from build123d import *

# Parameters (mm, degrees)
SKETCH1_R           = 1.5
BOSS_EXTRUDE2_DEPTH = 3.175


with BuildPart() as part:
    # Sketch1 → Boss-Extrude2 (new body)
    with BuildSketch(Plane(origin=(0, 0, 0), x_dir=(1, 0, 0), z_dir=(0, 1, 0))):
        with BuildLine():
            ThreePointArc((35.49727084, -66.067721036), (0, 75), (-35.49727084, -66.067721036))
            ThreePointArc((-35.49727084, -66.067721036), (-33.357679643, -66.33740492), (-31.589980006, -65.102164912))
            ThreePointArc((-31.589980006, -65.102164912), (0, -48.302004425), (31.589980006, -65.102164912))
            ThreePointArc((31.589980006, -65.102164912), (33.357679643, -66.33740492), (35.49727084, -66.067721036))
        make_face()
        with Locations((-13.608916499, -21.183093811)):
            Circle(SKETCH1_R, mode=Mode.SUBTRACT)
        with Locations((-46.011477091, 28.075890486)):
            Circle(SKETCH1_R, mode=Mode.SUBTRACT)
        with Locations((13.608916499, -21.183093811)):
            Circle(SKETCH1_R, mode=Mode.SUBTRACT)
        with Locations((23.852486199, -41.694616163)):
            Circle(SKETCH1_R, mode=Mode.SUBTRACT)
        with Locations((-42.910067426, 11.1)):
            Circle(SKETCH1_R, mode=Mode.SUBTRACT)
        with Locations((-42.910067426, -11.1)):
            Circle(SKETCH1_R, mode=Mode.SUBTRACT)
        with Locations((-11.160067426, -11.1)):
            Circle(SKETCH1_R, mode=Mode.SUBTRACT)
        with Locations((-11.160067426, 11.1)):
            Circle(SKETCH1_R, mode=Mode.SUBTRACT)
        with Locations((11.160067426, 11.1)):
            Circle(SKETCH1_R, mode=Mode.SUBTRACT)
        with Locations((11.160067426, -11.1)):
            Circle(SKETCH1_R, mode=Mode.SUBTRACT)
        with Locations((42.910067426, -11.1)):
            Circle(SKETCH1_R, mode=Mode.SUBTRACT)
        with Locations((42.910067426, 11.1)):
            Circle(SKETCH1_R, mode=Mode.SUBTRACT)
        with Locations((-23.852486199, -41.694616163)):
            Circle(SKETCH1_R, mode=Mode.SUBTRACT)
        with Locations((19.397913834, 18.186588214)):
            Circle(SKETCH1_R, mode=Mode.SUBTRACT)
        with Locations((-40.277379234, -25.14022965)):
            Circle(SKETCH1_R, mode=Mode.SUBTRACT)
        with Locations((40.277379234, -25.14022965)):
            Circle(SKETCH1_R, mode=Mode.SUBTRACT)
        with Locations((-22.416161975, 64.096715224)):
            Circle(SKETCH1_R, mode=Mode.SUBTRACT)
        with Locations((22.416161975, 64.096715224)):
            Circle(SKETCH1_R, mode=Mode.SUBTRACT)
        with Locations((26.163250867, 37.1696126)):
            Circle(SKETCH1_R, mode=Mode.SUBTRACT)
        with Locations((46.011477091, 28.075890486)):
            Circle(SKETCH1_R, mode=Mode.SUBTRACT)
        with Locations((10.027203595, 39.91869143)):
            Circle(SKETCH1_R, mode=Mode.SUBTRACT)
        with Locations((0, -39.659190322)):
            Circle(SKETCH1_R, mode=Mode.SUBTRACT)
        with Locations((-10.027203595, 39.91869143)):
            Circle(SKETCH1_R, mode=Mode.SUBTRACT)
        with Locations((-34.69516474, -58.122990171)):
            Circle(SKETCH1_R, mode=Mode.SUBTRACT)
        with Locations((-34.69516474, 58.122990171)):
            Circle(SKETCH1_R, mode=Mode.SUBTRACT)
        with Locations((34.69516474, -58.122990171)):
            Circle(SKETCH1_R, mode=Mode.SUBTRACT)
        with Locations((0, 15.543589551)):
            Circle(SKETCH1_R, mode=Mode.SUBTRACT)
        with Locations((-26.163250867, 37.1696126)):
            Circle(SKETCH1_R, mode=Mode.SUBTRACT)
        with Locations((-19.397913834, 18.186588214)):
            Circle(SKETCH1_R, mode=Mode.SUBTRACT)
        with Locations((34.69516474, 58.122990171)):
            Circle(SKETCH1_R, mode=Mode.SUBTRACT)
        with BuildLine():
            Line((53.410067426, -34), (53.410067426, 34))
            ThreePointArc((53.410067426, 34), (53.556514035, 34.353553391), (53.910067426, 34.5))
            Line((53.910067426, 34.5), (63.910067426, 34.5))
            ThreePointArc((63.910067426, 34.5), (64.263620817, 34.353553391), (64.410067426, 34))
            Line((64.410067426, 34), (64.410067426, -34))
            ThreePointArc((64.410067426, -34), (64.263620817, -34.353553391), (63.910067426, -34.5))
            Line((63.910067426, -34.5), (53.910067426, -34.5))
            ThreePointArc((53.910067426, -34.5), (53.556514035, -34.353553391), (53.410067426, -34))
        make_face(mode=Mode.SUBTRACT)
        with BuildLine():
            Line((-63.910067426, -34.5), (-53.910067426, -34.5))
            ThreePointArc((-53.910067426, -34.5), (-53.556514035, -34.353553391), (-53.410067426, -34))
            Line((-53.410067426, -34), (-53.410067426, 34))
            ThreePointArc((-53.410067426, 34), (-53.556514035, 34.353553391), (-53.910067426, 34.5))
            Line((-53.910067426, 34.5), (-63.910067426, 34.5))
            ThreePointArc((-63.910067426, 34.5), (-64.263620817, 34.353553391), (-64.410067426, 34))
            Line((-64.410067426, 34), (-64.410067426, -34))
            ThreePointArc((-64.410067426, -34), (-64.263620817, -34.353553391), (-63.910067426, -34.5))
        make_face(mode=Mode.SUBTRACT)
        with BuildLine():
            ThreePointArc((-5.853899988, 64.744946271), (0.003726822, 68.153564176), (5.857575472, 64.738461857))
            ThreePointArc((5.857575472, 64.738461857), (10.16, 61.422565207), (5.857575472, 58.106668557))
            ThreePointArc((5.857575472, 58.106668557), (0.003726822, 54.691566239), (-5.853899988, 58.100184144))
            ThreePointArc((-5.853899988, 58.100184144), (-10.167207264, 61.422565207), (-5.853899988, 64.744946271))
        make_face(mode=Mode.SUBTRACT)
    extrude(amount=BOSS_EXTRUDE2_DEPTH)


solid = part.part
Check sheet for the modelled part. Datum: model origin and axes. Units: mm. A direction names the side the tool comes from. Round coordinates to 2 decimals unless told otherwise and drop trailing zeros. Order: outer loops, then holes, each group sorted by start corner. A loop starts at its lowest first (then second) coordinate and runs counter-clockwise, first axis right, second up.
(1) Go/stop test with flat-tipped pins: P1, Ø1, axis at y = 0.5, z = -12.5, coming from the -X side; P2, Ø1.6, axis at y = 2.5, z = -13, coming from the +X side; P3, Ø1, axis at x = 53, y = 1, coming from the +Z side. Record where each tip stops, or that it passes through.
(2) Access from +Z, -Z, +X, -X, +Y, -Y to the whole of each face (thin tool, end or side, straight path). Record for faces 1 (the cylindrical face through (-0.096, 1.565, -68.153)), 2 (the cylindrical face through (-0.521, 1.565, 48.306)).
(3) Cross-section at D-D, the plane y = 1. State how many separate pieces and enclosed holes the cut face has, and give its area (3 significant figures).
(4) Cross-section at C-C, the plane z = 32. Enter the section's corners in (x, y) (3 decimals).
(5) Draft check along X on faces 3 (the flat face through (-1, 0, -5)), 4 (the cylindrical face through (-10.166, 1.565, -61.335)), 5 (the cylindrical face through (2.78, 1.57, -74.95)). Enter one of: pulls with the +X half, pulls with the -X half, needs draft (parallel to the pull), parting line crosses it, or undercut.
(6) Scan lines: probe 1 along X at (y, z) = (3.05, -9); probe 2 along X at (y, z) = (1.8, -2.5); probe 3 along X at (y, z) = (1.1, -59). Record each from-to range of solid material in increasing order.
(7) Cross-section at A-A, the plane z = 0. Enter the section's corners in (x, y) (3 decimals), and give its area (3 significant figures).
(8) Cross-section at B-B, the plane x = -56. Enter the section's corners in (y, z) (3 decimals).
Check sheet entries:
1. P1: stops at x = -74.03
1. P2: stops at x = 74
1. P3: stops at z = 53.56
2. face 1: +Y, -Y
2. face 2: +Z, +Y, -Y
3. separate pieces: 1
3. enclosed holes: 33
3. area: 14,500 mm2
4. outline: (-67.831, 0) - (-64.41, 0) - (-64.41, 3.175) - (-67.831, 3.175) - close; (-53.41, 0) - (53.41, 0) - (53.41, 3.175) - (-53.41, 3.175) - close; (64.41, 0) - (67.831, 0) - (67.831, 3.175) - (64.41, 3.175) - close
5. face 3: needs draft
5. face 4: undercut
5. face 5: parting line crosses it
6. probe 1: x = -74.46 to -64.41, -53.41 to 53.41, 64.41 to 74.46
6. probe 2: x = -74.96 to -64.41, -53.41 to 53.41, 64.41 to 74.96
6. probe 3: x = -46.3 to -35.91, -33.48 to -9.17, 9.16 to 33.48, 35.91 to 46.3
7. outline: (-75, 0) - (-64.41, 0) - (-64.41, 3.175) - (-75, 3.175) - close; (-53.41, 0) - (53.41, 0) - (53.41, 3.175) - (-53.41, 3.175) - close; (64.41, 0) - (75, 0) - (75, 3.175) - (64.41, 3.175) - close
7. area: 406 mm2
8. outline: (0, -49.89) - (3.175, -49.89) - (3.175, -34.5) - (0, -34.5) - close; (0, 34.5) - (3.175, 34.5) - (3.175, 49.89) - (0, 49.89) - close
